Autodesk Inventor part; units mm, degrees
ref_plane "YZ Plane" through (0, 0, 0) normal (1, 0, 0) x (0, 1, 0)
ref_plane "XZ Plane" through (0, 0, 0) normal (0, 1, 0) x (-1, 0, 0)
ref_plane "XY Plane" through (0, 0, 0) normal (0, 0, 1) x (1, 0, 0)
sketch "Эскиз1" plane through (0, 0, 0) normal (0, 1, 0) x (-1, 0, 0)
  line L0 (0, 0) -> (40, 0)
  line L1 (40, 0) -> (40, -60)
  line L2 (40, -60) -> (0, -60)
  line L3 (0, -60) -> (0, 0)
  line L4 (37, -12) -> (21, -12)
  line L5 (21, -12) -> (21, -28)
  line L6 (21, -28) -> (37, -28)
  line L7 (37, -28) -> (37, -12)
  line L8 (37, -32) -> (21, -32)
  line L9 (21, -32) -> (21, -48)
  line L10 (21, -48) -> (37, -48)
  line L11 (37, -48) -> (37, -32)
  line L12 (0, -21) -> (18, -21)
  line L13 (18, -21) -> (18, -39)
  line L14 (18, -39) -> (0, -39)
  line L15 (0, -39) -> (0, -21)
  circle A0 centre (2, -2) radius 1.5
  circle A1 centre (2, -58) radius 1.5
  circle A2 centre (38, -2) radius 1.5
  circle A3 centre (38, -58) radius 1.5
  point P0 (0, -39)
  dimension "d0" = 40
  dimension "d1" = 60
  dimension "d2" = 16
  dimension "d3" = 16
  dimension "d4" = 3
  dimension "d5" = 12
  dimension "d6" = 16
  dimension "d7" = 16
  dimension "d8" = 4
  dimension "d9" = 3
  dimension "d10" = 18
  dimension "d11" = 18
  dimension "d12" = 21
  dimension "d13" = 3
  dimension "d14" = 2
  dimension "d15" = 2
  dimension "d18" = 56
  dimension "d21" = 36
extrude "Выдавливание1" add sketch "Эскиз1" along normal blind 1.6 contours L0 L1 L2 L3 L14 L13 L12
extrude "Выдавливание2" add sketch "Эскиз1" along normal blind 11.6 contours L7 L6 L5 L4 | L11 L10 L9 L8
extrude "Выдавливание3" add sketch "Эскиз1" along normal blind 3.6 contours L12 L13 L14 L3
properties part number "plate"
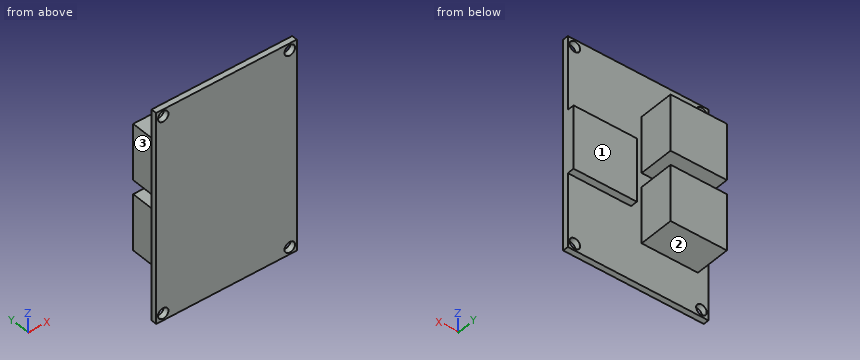
Geometry check sheet. Reference: the model listing, model coordinates, mm. Face numbers are marked on the shaded views. A direction names the side the tool comes from. Coordinates: 2 decimals unless noted, no trailing zeros. Write each loop counter-clockwise with the first axis right and the second up, starting at its lowest first coordinate (ties: lowest second). Pieces come first, ordered by that corner, then holes. Notation, with made-up numbers: M 38.25,-8.75 L 64.25,-8.75 A32 cw 64.25,17.25 Z; hole C 62.25,-19 d1. An arc over 180 degrees is marked long. One line per item, written item: value. Start each with the question number.
(1) Sectioned sample at D-D, the plane z = -42. Enter the section's corners in (x, y).
(2) Sectioned sample at C-C, the plane z = -2. Enter the section's corners in (x, y).
(3) Depth check by flat-ended pin: pin 1 (1.8 mm diameter, centred on x = -2, z = -2, fed in from -Y); pin 2 (3 mm diameter, centred on y = 6, z = -37, fed in from -X); pin 3 (3 mm diameter, centred on x = -28, y = 7.5, fed in from -Z); pin 4 (3 mm diameter, centred on x = -29, y = 6.5, fed in from +Z). Enter the tip coordinate at first touch or a pass-through.
(4) Sectioned sample at B-B, the plane y = 5.5. Enter the section's corners in (x, z).
(5) Scan lines: line 1 along Z through (x, y) = (-2, 0.55); line 2 along Z through (x, y) = (-25, 1.75); line 3 along Y through (x, z) = (-38, -47). Record each from-to range of solid material in increasing order. Write a range as [from, to].
(6) Tool access check on the marked faces 1, 2 and 3. Record the directions out of +Z, -Z, +X, -X, +Y, -Y that give a thin tool (end or side, any length) a straight path to the whole face; none if there is none.
(7) Sectioned sample at A-A, the plane x = -38. Enter the section's corners in (y, z).
Filled sheet:
1. outline: M -40,0 L 0,0 L 0,1.6 L -21,1.6 L -21,11.6 L -37,11.6 L -37,1.6 L -40,1.6 Z
2. outline: M -40,0 L -39.5,0 L -39.5,1.6 L -40,1.6 Z; M -36.5,0 L -3.5,0 L -3.5,1.6 L -36.5,1.6 Z; M -0.5,0 L 0,0 L 0,1.6 L -0.5,1.6 Z
3. pin 1: through
3. pin 2: x = -37
3. pin 3: z = -48
3. pin 4: z = -12
4. outline: M -37,-48 L -21,-48 L -21,-32 L -37,-32 Z; M -37,-28 L -21,-28 L -21,-12 L -37,-12 Z
5. line 1: [-60, -59.5], [-56.5, -3.5], [-0.5, 0]
5. line 2: [-48, -32], [-28, -12]
5. line 3: [0, 1.6]
6. face 1: +Z, -Z, +X, +Y
6. face 2: -Z, +X, -X, +Y
6. face 3: +Z, -Z, -X, +Y
7. outline: M 0,-60 L 1.6,-60 L 1.6,-59.5 L 0,-59.5 Z; M 0,-56.5 L 1.6,-56.5 L 1.6,-3.5 L 0,-3.5 Z; M 0,-0.5 L 1.6,-0.5 L 1.6,0 L 0,0 Z
